```python
from build123d import *

# Parameters (mm, degrees)
SKETCH1_R             = 11.43
SKETCH1_R_2           = 8.255
BOSS_EXTRUDE1_DEPTH   = 2.54
F_2_56_TAPPED_HOLE1_D = 1.778


with BuildPart() as part:
    # Sketch1 → Boss-Extrude1 (new body)
    with BuildSketch(Plane.XY):
        Circle(SKETCH1_R)
        Circle(SKETCH1_R_2, mode=Mode.SUBTRACT)
    extrude(amount=BOSS_EXTRUDE1_DEPTH)

    # #2-56 Tapped Hole1 (through all)
    with Locations(Plane.XY.offset(2.54)):
        with Locations((0, 9.525)):
            f_2_56_tapped_hole1 = Hole(F_2_56_TAPPED_HOLE1_D / 2)

    # Mirror1: #2-56 Tapped Hole1 across plane
    add(f_2_56_tapped_hole1.mirror(Plane.ZX), mode=Mode.SUBTRACT)


solid = part.part
```
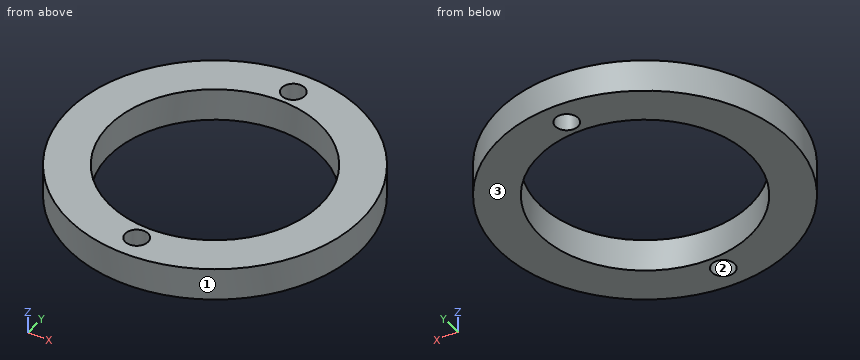
Could you check a few things on this model? Use its own coordinates, in mm. Face numbers are marked on the shaded views. Round coordinates to 2 decimals unless told otherwise and drop trailing zeros. Loops run counter-clockwise (first coordinate to the right, second up) from the corner with the lowest first, then second, coordinate; pieces in that order, holes last. Notation, with made-up numbers: M -37.75,-7 L -26.75,-7 A25 cw -26.75,14 Z; hole C 24,19.25 d2. An arc over 180 degrees is marked long. Write item = value, one per line.
1. Thinking about a two-plate mould opening in Y: for the marked faces 1, 2 and 3, which applies, +Y half, -Y half, draft (parallel to the pull), parting line (faces both ways), or undercut?
Results below:
face_1 = parting line
face_2 = undercut
face_3 = draft
2. I want a section at A-A, the plane x = 0. Write out the boundary of the cut face in (y, z) (3 decimals), and give its area (3 significant figures).
Results below:
outline = M -11.43,0 L -10.414,0 L -10.414,2.54 L -11.43,2.54 Z; M -8.636,0 L -8.255,0 L -8.255,2.54 L -8.636,2.54 Z; M 8.255,0 L 8.636,0 L 8.636,2.54 L 8.255,2.54 Z; M 10.414,0 L 11.43,0 L 11.43,2.54 L 10.414,2.54 Z
area = 7.10 mm²
3. I want a section at D-D, the plane z = 1.5. Write out the boundary of the cut face in (x, y) (3 decimals), and give its area (3 significant figures).
Results below:
outline = C 0,0 d22.86; hole C 0,0 d16.51; hole C 0,-9.525 d1.778; hole C 0,9.525 d1.778
area = 191 mm²
4. I need wall thicknesses on probe 1 along Y at (x, z) = (0, 1.1) (3 decimals); probe 2 along Y at (x, z) = (0.25, 1.05); probe 3 along X at (y, z) = (-1.5, 1.85). Which ranges of each line are inside material? Lowest first, please.
Results below:
probe_1 = -11.43 to -10.414, -8.636 to -8.255, 8.255 to 8.636, 10.414 to 11.43
probe_2 = -11.43 to -10.38, -8.67 to -8.25, 8.25 to 8.67, 10.38 to 11.43
probe_3 = -11.33 to -8.12, 8.12 to 11.33
5. I want a section at B-B, the plane y = 0. Write out the boundary of the cut face in (x, z) (3 decimals), and give its area (3 significant figures).
Results below:
outline = M -11.43,0 L -8.255,0 L -8.255,2.54 L -11.43,2.54 Z; M 8.255,0 L 11.43,0 L 11.43,2.54 L 8.255,2.54 Z
area = 16.1 mm²
6. Will these pins go through, and if not, where does the flat tip stop? P1, Ø2.5, axis at x = 0, y = -9.525, coming from the -Z side; P2, Ø1.4, axis at x = 0, y = 9.525, coming from the -Z side; P3, Ø1.5, axis at x = 9, z = 2, coming from the -Y side.
Results below:
P1 = 0
P2 = through
P3 = -7.91
7. I want a section at C-C, the plane x = 7.25. Write out the boundary of the cut face in (y, z).
Results below:
outline = M -8.84,0 L -3.95,0 L -3.95,2.54 L -8.84,2.54 Z; M 3.95,0 L 8.84,0 L 8.84,2.54 L 3.95,2.54 Z
